```python
from build123d import *

# Parameters (mm, degrees)
BOSS_EXTRUDE1_DEPTH = 50
SKETCH3_R           = 0.55
CUT_EXTRUDE1_DEPTH  = 3
SKETCH4_R           = 1.75
CUT_EXTRUDE2_DEPTH  = 26


with BuildPart() as part:
    # Sketch1 → Boss-Extrude1 (new body)
    with BuildSketch(Plane.XY):
        Polygon((0, 0), (0, 25), (30, 25), (30, 14.553417219), (23, 14.553417219), (23, 22), (5, 22), (5, 3), (23, 3), (23, 9.833225485), (30, 9.833225485), (30, 0), align=None)
    extrude(amount=BOSS_EXTRUDE1_DEPTH)

    # Sketch3 → Cut-Extrude1 (cut)
    with BuildSketch(Plane.ZY):
        Polygon((4.919472148, 16.056705519), (21.919472148, 16.056705519), (21.919472148, 24.056705519), (27.919472148, 24.056705519), (27.919472148, 16.056705519), (42.919472148, 16.056705519), (42.919472148, 9.056705519), (27.919472148, 9.056705519), (27.919472148, 1.056705519), (21.919472148, 1.056705519), (21.919472148, 9.056705519), (4.919472148, 9.056705519), align=None)
        with Locations((40.25, 12.520312642)):
            Circle(SKETCH3_R, mode=Mode.SUBTRACT)
        with Locations((8.980224058, 12.520312642)):
            Circle(SKETCH3_R, mode=Mode.SUBTRACT)
    extrude(amount=-CUT_EXTRUDE1_DEPTH, mode=Mode.SUBTRACT)

    # Sketch4 → Cut-Extrude2 (cut)
    with BuildSketch(Plane(origin=(0, 25, 0), x_dir=(1, 0, 0), z_dir=(0, 1, 0))):
        with Locations((27.668171427, -27.18874166)):
            Circle(SKETCH4_R)
    extrude(amount=-CUT_EXTRUDE2_DEPTH, mode=Mode.SUBTRACT)


solid = part.part
```
The model under review builds one solid part; all positions refer to its coordinate system, in mm. A direction names the side the tool comes from. Give positions to 0.01 mm unless a question says otherwise; leave off trailing zeros. Write each loop counter-clockwise with the first axis right and the second up, starting at its lowest first coordinate (ties: lowest second). Pieces come first, ordered by that corner, then holes. Notation, with made-up numbers: (-18.75, 77.25) -> (-8.75, 77.25) arc R15 cw to (-8.75, 98.25) -> close; hole circle Ø3 at (86, 31.25). An arc over 180 degrees is marked (long way). Answer in a Markdown table with one row per item.
1) For L1, parallel to X at y = 15.5, z = 17; L2, parallel to Y at x = 9.5, z = 34.5; L3, parallel to X at y = 19.5, z = 21, list the stretches that pass through material, from the lowest coordinate up. Write a range as [from, to].
Worked answers:
| item | result |
|---|---|
| L1 | [3, 5], [23, 30] |
| L2 | [0, 3], [22, 25] |
| L3 | [0, 5], [23, 30] |
2) Tool access review of faces 4 (the flat face through (25, 15, 50)), 5 (the flat face through (23, 6, 25)), 6 (the flat face through (1, 24.057, 25)): name each direction out of +Z, -Z, +X, -X, +Y, -Y from which nothing blocks a thin tool from reaching the whole face with its end or side.
Worked answers:
| item | result |
|---|---|
| face 4 | +Z, +X, -X, +Y, -Y |
| face 5 | +Z, -Z |
| face 6 | -X |
3) Add section A-A on x = 14.25. State the section outline as (y, z) points.
Worked answers:
| item | result |
|---|---|
| outline | (0, 0) -> (3, 0) -> (3, 50) -> (0, 50) -> close; (22, 0) -> (25, 0) -> (25, 50) -> (22, 50) -> close |
4) Add section C-C on z = 18.5. State the section outline as (x, y) points, plus the area to 3 significant figures.
Worked answers:
| item | result |
|---|---|
| outline | (0, 0) -> (30, 0) -> (30, 9.83) -> (23, 9.83) -> (23, 3) -> (5, 3) -> (5, 22) -> (23, 22) -> (23, 14.55) -> (30, 14.55) -> (30, 25) -> (0, 25) -> (0, 16.06) -> (3, 16.06) -> (3, 9.06) -> (0, 9.06) -> close |
| area | 354 mm² |
5) Add section B-B on y = 16.75. State the section outline as (x, z) points, plus the area to 3 significant figures.
Worked answers:
| item | result |
|---|---|
| outline | (0, 0) -> (5, 0) -> (5, 50) -> (0, 50) -> (0, 27.92) -> (3, 27.92) -> (3, 21.92) -> (0, 21.92) -> close; (23, 0) -> (30, 0) -> (30, 50) -> (23, 50) -> close; hole circle Ø3.5 at (27.67, 27.19) |
| area | 572 mm² |
6) Mouldability with a two-part tool opening along Y and no side actions: class faces 1 (the flat face through (15, 0, 25)), 2 (the flat face through (25, 15, 0)), 3 (the flat face through (14, 3, 25)) as +Y half, -Y half, draft (parallel to the pull), parting line (faces both ways), or undercut.
Worked answers:
| item | result |
|---|---|
| face 1 | -Y half |
| face 2 | draft |
| face 3 | undercut |
7) Add section D-D on y = 23. State the section outline as (x, z) points, plus the area to 3 significant figures.
Worked answers:
| item | result |
|---|---|
| outline | (0, 0) -> (30, 0) -> (30, 50) -> (0, 50) -> (0, 27.92) -> (3, 27.92) -> (3, 21.92) -> (0, 21.92) -> close; hole circle Ø3.5 at (27.67, 27.19) |
| area | 1,470 mm² |
